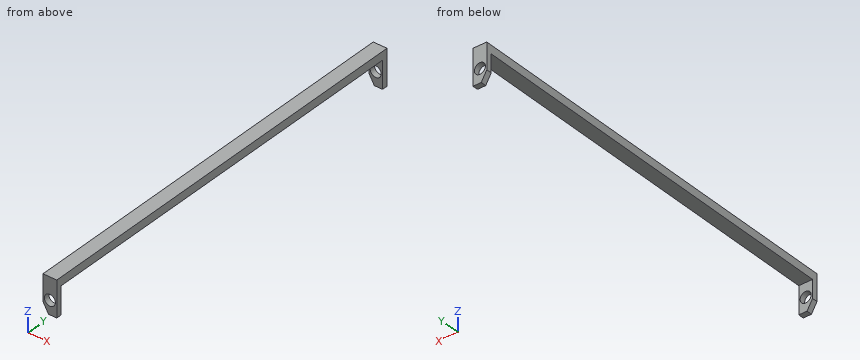
```python
from build123d import *

# Parameters (mm, degrees)
ESQUISSE1_R        = 2
BOSS_EXTRU_1_DEPTH = 2
ESQUISSE2_W        = 5
ESQUISSE2_H        = 3
BOSS_EXTRU_2_DEPTH = 144.52
ESQUISSE3_R        = 2
BOSS_EXTRU_3_DEPTH = 2


with BuildPart() as part:
    # Esquisse1 → Boss.-Extru.1 (new body)
    with BuildSketch(Plane(origin=(0, 0, 0), x_dir=(1, 0, 0), z_dir=(0, 1, 0))):
        Polygon((2.01, 10), (0, 6.52), (0, 0), (0, -3), (5, -3), (5, 0), (5, 10), align=None)
        with Locations(Location((2.5, 5, 0), (0, 0, 270))):
            Circle(ESQUISSE1_R, mode=Mode.SUBTRACT)
    extrude(amount=BOSS_EXTRU_1_DEPTH)

    # Esquisse2 → Boss.-Extru.2 (add)
    with BuildSketch(Plane(origin=(0, 2, 0), x_dir=(1, 0, 0), z_dir=(0, 1, 0))):
        with Locations((2.5, -1.5)):
            Rectangle(ESQUISSE2_W, ESQUISSE2_H)
    extrude(amount=BOSS_EXTRU_2_DEPTH)

    # Esquisse3 → Boss.-Extru.3 (add)
    with BuildSketch(Plane(origin=(0, 146.52, 0), x_dir=(1, 0, 0), z_dir=(0, 1, 0))):
        Polygon((2.01, 10), (0, 6.52), (0, -3), (5, -3), (5, 10), align=None)
        with Locations(Location((2.5, 5, 0), (0, 0, 270))):
            Circle(ESQUISSE3_R, mode=Mode.SUBTRACT)
    extrude(amount=BOSS_EXTRU_3_DEPTH)


solid = part.part
```
Source: CAD feature listing. Evaluate the final solid. Frame: model axes, mm. Give positions to 0.01 mm unless a question says otherwise; leave off trailing zeros. Loops run counter-clockwise (first coordinate to the right, second up) from the corner with the lowest first, then second, coordinate; pieces in that order, holes last. Notation, with made-up numbers: (25, 65) - (74, 65) arc R19 ccw to (74, 71) - close; hole circle Ø8 at (77.25, 68). An arc over 180 degrees is marked (long way). Use CSV: the item, a comma, the result in double quotes. Start each with the question number.
1. Ray query, L1, parallel to X at y = 1.5, z = -5; L2, parallel to Y at x = 3.4, z = -8; L3, parallel to Z at x = 3.8, y = 100. Return the intervals inside material, ascending.
2. Section A-A (z = -1.75). Output: boundary loops of the cut face in (x, y).
3. Section B-B (y = 116.5). Output: boundary loops of the cut face in (x, z), then the cut area to 3 significant figures.
4. Pin query (flat end, axial travel): pin 1 (1 mm diameter, centred on x = 2.5, y = 30, fed in from -Z); pin 2 (1 mm diameter, centred on x = 2.5, z = -8, fed in from -Y). Return the tip coordinate at first contact, or that it passes through.
Response:
1,L1,"0 to 0.5, 4.5 to 5"
1,L2,"0 to 2, 146.52 to 148.52"
1,L3,"0 to 3"
2,outline,"(0, 0) - (5, 0) - (5, 2) - (0, 2) - close; (0, 146.52) - (5, 146.52) - (5, 148.52) - (0, 148.52) - close"
3,outline,"(0, 0) - (5, 0) - (5, 3) - (0, 3) - close"
3,area,"15.0 mm²"
4,pin 1,"z = 0"
4,pin 2,"y = 0"
